from build123d import *

# Parameters (mm, degrees)
ESQUISSE2_R             = 35
BOSS_EXTRU_1_DEPTH      = 40
CONG_1_R                = 10
ESQUISSE3_R             = 20
ENL_V_MAT_EXTRU_1_DEPTH = 30
ESQUISSE7_R             = 25
ENL_V_MAT_EXTRU_3_DEPTH = 3
ESQUISSE8_R             = 10
ENL_V_MAT_EXTRU_4_DEPTH = 45
ESQUISSE4_R             = 2.5
ENL_V_MAT_EXTRU_5_DEPTH = 30
ESQUISSE9_R             = 1.5
ENL_V_MAT_EXTRU_6_DEPTH = 16


with BuildPart() as part:
    # Esquisse2 → Boss.-Extru.1 (new body)
    with BuildSketch(Plane(origin=(0, 0, 0), x_dir=(1, 0, 0), z_dir=(0, 1, 0))):
        with Locations(Location((0, 0, 0), (0, 0, 270))):
            Circle(ESQUISSE2_R)
    extrude(amount=BOSS_EXTRU_1_DEPTH)

    # Congé1
    cong_1_edges = [part.edges().sort_by_distance(p)[0] for p in [
        (0, 40, -35),
    ]]
    fillet(cong_1_edges, radius=CONG_1_R)

    # Esquisse3 → Enlèv. mat.-Extru.1 (cut)
    with BuildSketch(Plane.XZ):
        with Locations(Location((0, 0, 0), (0, 0, 270))):
            Circle(ESQUISSE3_R)
    extrude(amount=-ENL_V_MAT_EXTRU_1_DEPTH, mode=Mode.SUBTRACT)

    # Esquisse7 → Enlèv. mat.-Extru.3 (cut)
    with BuildSketch(Plane(origin=(0, 40, 0), x_dir=(1, 0, 0), z_dir=(0, 1, 0))):
        with Locations(Location((0, 0, 0), (0, 0, 270))):
            Circle(ESQUISSE7_R)
    extrude(amount=-ENL_V_MAT_EXTRU_3_DEPTH, mode=Mode.SUBTRACT)

    # Esquisse8 → Enlèv. mat.-Extru.4 (cut)
    with BuildSketch(Plane.XY):
        with Locations(Location((0, 15, 0), (0, 0, 180))):
            Circle(ESQUISSE8_R)
    extrude(amount=ENL_V_MAT_EXTRU_4_DEPTH, mode=Mode.SUBTRACT)

    # Esquisse4 → Enlèv. mat.-Extru.5 (cut)
    with BuildSketch(Plane.XZ):
        with Locations(Location((0, 25, 0), (0, 0, 270))):
            Circle(ESQUISSE4_R)
    extrude(amount=-ENL_V_MAT_EXTRU_5_DEPTH, mode=Mode.SUBTRACT)

    # Esquisse9 → Enlèv. mat.-Extru.6 (cut)
    with BuildSketch(Plane.XZ):
        with Locations(Location((-27.5, 0, 0), (0, 0, 270))):
            Circle(ESQUISSE9_R)
        with Locations(Location((27.5, 0, 0), (0, 0, 270))):
            Circle(ESQUISSE9_R)
    extrude(amount=-ENL_V_MAT_EXTRU_6_DEPTH, mode=Mode.SUBTRACT)


solid = part.part
Check sheet for the modelled part. Datum: model origin and axes. Units: mm. A direction names the side the tool comes from. Round coordinates to 2 decimals unless told otherwise and drop trailing zeros. Loops run counter-clockwise (first coordinate to the right, second up) from the corner with the lowest first, then second, coordinate; pieces in that order, holes last.
1. Sectioned sample at D-D on y = 31. Record the boundary of the cut face in (x, z), and give its area (3 significant figures).
2. Sectioned sample at B-B on y = 15. Record the boundary of the cut face in (x, z), and give its area (3 significant figures).
3. Sectioned sample at A-A on x = 0. Record the boundary of the cut face in (y, z).
4. Gauge pin test, flat ends, axial feed: pin 1 Ø10 at (y, z) = (18.5, 16) entering from +X; pin 2 Ø8 at (x, z) = (20.5, -27) entering from +Y; pin 3 Ø2.5 at (x, z) = (-27.5, 0) entering from +Y. Record the tip position at first contact, or that the pin passes through.
5. Scan lines: probe 1 along Y at (x, z) = (16.5, 2.5); probe 2 along X at (y, z) = (38.8, 0); probe 3 along X at (y, z) = (19, -12). Record each from-to range of solid material in increasing order.
6. Set-up check for faces 4 (the cylindrical face through (29, 8, 0)), 5 (the cylindrical face through (7.509, 38.521, 23.846)), 6 (the cylindrical face through (-9.237, 18.83, 26.036)): record each of +Z, -Z, +X, -X, +Y, -Y from which the full face is reachable in a straight line by a thin tool's end or side.
7. Sectioned sample at C-C on y = 38.5. Record the boundary of the cut face in (x, z).
8. Mould release check, pull along Z, two halves, no side actions. Record for faces 1 (the flat face through (-15, 0, 15)), 2 (the cylindrical face through (-21, 15, -28)), 3 (the cylindrical face through (6.007, 14.79, -19.076)): released by +Z, released by -Z, zero draft, split by the parting line, or undercut.
Recorded:
1. outline: circle Ø69.9 at (0, 0)
1. area: 3,840 mm2
2. outline: (-10, 17.32) - (-10, 33.54) arc R35 ccw (long way) to (10, 33.54) - (10, 17.32) arc R20 cw (long way) to start; hole circle Ø3 at (-27.5, 0); hole circle Ø3 at (27.5, 0)
2. area: 2,270 mm2
3. outline: (0, -35) - (30, -35) arc R10 ccw to (40, -25) - (37, -25) - (37, 25) - (40, 25) arc R10 ccw to (30, 35) - (25, 35) - (25, 27.5) - (30, 27.5) - (30, 22.5) - (25, 22.5) - (25, 20) - (30, 20) - (30, -20) - (0, -20) - close; (0, 20) - (5, 20) - (5, 22.5) - (0, 22.5) - close; (0, 27.5) - (5, 27.5) - (5, 35) - (0, 35) - close
4. pin 1: stops at x = 33.23
4. pin 2: stops at y = 38.72
4. pin 3: stops at y = 39.92
5. probe 1: y = 30 to 37
5. probe 2: x = -29.75 to -25, 25 to 29.75
5. probe 3: x = -32.88 to -16, 16 to 32.88
6. face 4: -Y
6. face 5: +Y
6. face 6: +Z
7. outline: circle Ø60.54 at (0, 0); hole circle Ø50 at (0, 0)
8. face 1: zero draft
8. face 2: split by the parting line
8. face 3: undercut
